Check sheet for the drawn part. Datum: minimum x, y, z corner. Units: mm. A direction names the side the tool comes from. Round coordinates to 2 decimals unless told otherwise and drop trailing zeros. Loops run counter-clockwise (first coordinate to the right, second up) from the corner with the lowest first, then second, coordinate; pieces in that order, holes last.
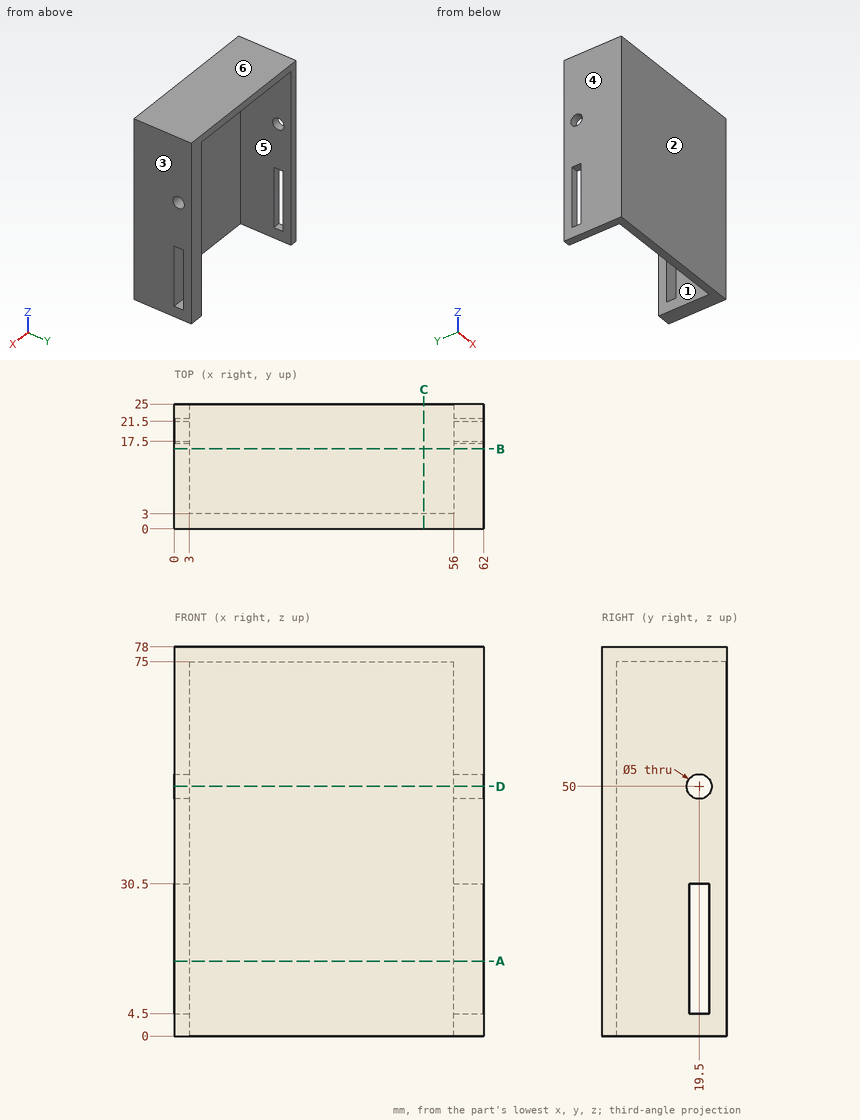
1. Release check for a two-part mould opening along X. For the marked faces 3, 4, 5 and 6 record: released by +X, released by -X, zero draft, split by the parting line, or undercut.
2. Section check A-A (z = 15). Enter the section's corners in (x, y).
3. Gauge pin test, flat ends, axial feed: P1, Ø4.5, axis at x = 60, y = 19, coming from the -Z side; P2, Ø3, axis at y = 19.5, z = 50, coming from the +X side; P3, Ø10, axis at x = 18.5, y = 10.5, coming from the -Z side; P4, Ø16, axis at x = 27.5, z = 45, coming from the +Y side. Record the tip position at first contact, or that the pin passes through.
4. Tool access check on the marked faces 1 and 2. Record the directions out of +Z, -Z, +X, -X, +Y, -Y that give a thin tool (end or side, any length) a straight path to the whole face; none if there is none.
5. Section check D-D (z = 50). Enter the section's corners in (x, y), then the cut area to 3 significant figures.
6. Section check B-B (y = 16). Enter the section's corners in (x, z), then the cut area to 3 significant figures.
7. Section check C-C (x = 50). Enter the section's corners in (y, z), then the cut area to 3 significant figures.
8. Scan lines: L1, parallel to Y at x = 60, z = 50; L2, parallel to X at y = 7, z = 4.5; L3, parallel to Y at x = 18, z = 45. Record each from-to range of solid material in increasing order.
Taken from the geometry:
1. face 3: released by +X
1. face 4: released by -X
1. face 5: undercut
1. face 6: zero draft
2. outline: (0, 0) - (62, 0) - (62, 17.5) - (56, 17.5) - (56, 3) - (3, 3) - (3, 17.5) - (0, 17.5) - close; (0, 21.5) - (3, 21.5) - (3, 25) - (0, 25) - close; (56, 21.5) - (62, 21.5) - (62, 25) - (56, 25) - close
3. P1: stops at z = 0
3. P2: passes through
3. P3: stops at z = 75
3. P4: stops at y = 3
4. face 1: -Z, +Y
4. face 2: +Z, -Z, +X, -X, -Y
5. outline: (0, 0) - (62, 0) - (62, 17) - (56, 17) - (56, 3) - (3, 3) - (3, 17) - (0, 17) - close; (0, 22) - (3, 22) - (3, 25) - (0, 25) - close; (56, 22) - (62, 22) - (62, 25) - (56, 25) - close
5. area: 339 mm2
6. outline: (0, 0) - (3, 0) - (3, 75) - (56, 75) - (56, 0) - (62, 0) - (62, 78) - (0, 78) - close
6. area: 861 mm2
7. outline: (0, 0) - (3, 0) - (3, 75) - (25, 75) - (25, 78) - (0, 78) - close
7. area: 300 mm2
8. L1: y = 0 to 17, 22 to 25
8. L2: x = 0 to 3, 56 to 62
8. L3: y = 0 to 3
